Read the model definition and answer for the solid it produces. Units are mm, in the model's axes. Face numbers are marked on the shaded views. A direction names the side the tool comes from. Coordinates: 2 decimals unless noted, no trailing zeros. Write each loop counter-clockwise with the first axis right and the second up, starting at its lowest first coordinate (ties: lowest second). Pieces come first, ordered by that corner, then holes.
from build123d import *

# Parameters (mm, degrees)
F1_DEPTH = 10


with BuildPart() as f1:
    # F0 (on Right) → F1 (new body)
    with BuildSketch(Plane.YZ):
        with BuildLine():
            Line((-21.091432, 25.457158), (-30, 30))
            Line((-30, 30), (-30, 20))
            ThreePointArc((-30, 20), (-18.027756, 5.458365), (0, 0))
            Line((0, 0), (20, 0))
            ThreePointArc((20, 0), (45, -8.333333), (60, -30))
            Line((60, -30), (70, -30))
            Line((70, -30), (70, -20))
            Line((70, -20), (70, 10))
            Line((70, 10), (70, 20))
            Line((70, 20), (1.622777, 20))
            ThreePointArc((1.622777, 20), (-10.057504, 21.383428), (-21.091432, 25.457158))
        make_face()
        Polygon((90, 20), (70, 20), (70, 10), (80, 10), (80, 0), (90, 0), align=None)
        Polygon((80, -20), (70, -20), (70, -30), (90, -30), (90, -10), (80, -10), align=None)
    extrude(amount=F1_DEPTH)


solid = f1.part
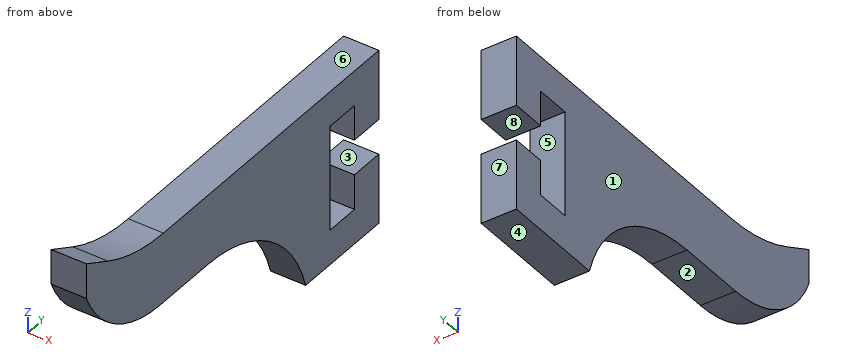
Item 1: Find the intervals of material crossed by probe 1 along Z at (x, y) = (1, 79.5); probe 2 along Y at (x, z) = (9.75, -14.5); probe 3 along Y at (x, z) = (3.75, 4), in increasing order.
Item 2: The part is cut by section B-B (x = 3.5). Give the vertices of the cut face in (y, z).
Item 3: The part is cut by section C-C (y = 8.5). Give the vertices of the cut face in (x, z).
Item 4: For the marked faces 4, 5, 6, 7 and 8, determine the directions among +Z, -Z, +X, -X, +Y, -Y from which every point of the face is accessible in a straight line to the end or side of a thin tool.
Item 5: Given pin 1 (5 mm diameter, centred on x = 5, z = 4, fed in from -Y); pin 2 (3 mm diameter, centred on x = 7, y = 67.5, fed in from +Z); pin 3 (2 mm diameter, centred on x = 5, y = -6, fed in from +Z), each flat-ended and moving along its own axis, determine where each tip first touches the part or whether it passes through.
Item 6: The part is cut by section A-A (z = 3). Give the vertices of the cut face in (x, y), and give its area (3 significant figures).
Item 7: The part is cut by section D-D (z = 16). Give the vertices of the cut face in (x, y), and give its area (3 significant figures).
Item 8: Determine the mould class of the marked faces 1, 2 and 3 for opening direction Z: +Z half, -Z half, draft (parallel to the pull), parting line (faces both ways), or undercut.
Answer:
1. probe 1: z = -30 to -20, 10 to 20
1. probe 2: y = 51.59 to 70, 80 to 90
1. probe 3: y = -15.62 to 70, 80 to 90
2. outline: (-30, 20) arc R32.5 ccw to (0, 0) - (20, 0) arc R41.67 cw to (60, -30) - (90, -30) - (90, -10) - (80, -10) - (80, -20) - (70, -20) - (70, 10) - (80, 10) - (80, 0) - (90, 0) - (90, 20) - (1.62, 20) arc R50 cw to (-21.09, 25.46) - (-30, 30) - close
3. outline: (0, 0) - (10, 0) - (10, 20) - (0, 20) - close
4. face 4: -Z, +X, -X, +Y, -Y
4. face 5: +X, -X
4. face 6: +Z, +X, -X, +Y
4. face 7: +Z, -Z, +X, -X, +Y
4. face 8: +X, -X, +Y
5. pin 1: stops at y = -19.5
5. pin 2: stops at z = 20
5. pin 3: stops at z = 20.75
6. outline: (0, -13.64) - (10, -13.64) - (10, 70) - (0, 70) - close; (0, 80) - (10, 80) - (10, 90) - (0, 90) - close
6. area: 936 mm2
7. outline: (0, -28) - (10, -28) - (10, 90) - (0, 90) - close
7. area: 1,180 mm2
8. face 1: draft
8. face 2: -Z half
8. face 3: undercut
